from build123d import *

# Parameters (mm, degrees)
F0_W        = 31.75
F0_H        = 31.75
F1_DEPTH    = 6.35
F2_SIZE2    = 5.5380575658
F2_SIZE     = 6.6
F4_DEPTH    = 5.08
F5_T1_DEPTH = 36.3880046162
F5_T3_DEPTH = 36.3880046162


# Not quite as in the source:
# - a fillet or chamfer that OpenCascade refuses, or shapes differently, is made with other operations: its cross-section is extruded or revolved along the edge and cut away or added


with BuildPart() as f1:
    # F0 (on Top) → F1 (new body)
    with BuildSketch(Plane.XY):
        Rectangle(F0_W, F0_H)
    extrude(amount=F1_DEPTH)

    # F2
    f2_edges = [f1.edges().sort_by_distance(p)[0] for p in [
        (-15.875, 0, 6.35),
        (0, -15.875, 6.35),
        (15.875, 0, 6.35),
        (0, 15.875, 6.35),
    ]]
    f2_side = f1.faces().sort_by_distance((0, 0, 6.35))[0]
    chamfer(f2_edges, length=F2_SIZE, length2=F2_SIZE2, reference=f2_side)

    # F3 (on face) → F4 (cut)
    with BuildSketch(Plane.XY.offset(6.35)):
        with BuildLine():
            Line((9.25, -9.25), (9.25, 0))
            ThreePointArc((9.25, 0), (0, 9.25), (-9.25, 0))
            Line((-9.25, 0), (-9.25, -9.25))
            Line((-9.25, -9.25), (9.25, -9.25))
        make_face()
    extrude(amount=-F4_DEPTH, mode=Mode.SUBTRACT)

    # F5: fillet of radius 2 on 4 edges, made by hand

    # F5_s2 → F5_t1 (cut)
    with BuildSketch(Plane.YZ.offset(-18.1940023081)):
        with BuildLine():
            ThreePointArc((-15.875, 0), (-15.6643933238, 0.7771054734), (-15.1644164673, 1.4081928144))
            Line((-15.1644164673, 1.4081928144), (-15.875, 0.8119424342))
            Line((-15.875, 0.8119424342), (-15.875, 0))
        make_face()
        with BuildLine():
            ThreePointArc((15.875, 0), (15.6643933238, 0.7771054734), (15.1644164673, 1.4081928144))
            Line((15.1644164673, 1.4081928144), (15.875, 0.8119424342))
            Line((15.875, 0.8119424342), (15.875, 0))
        make_face()
    extrude(amount=F5_T1_DEPTH, mode=Mode.SUBTRACT)

    # F5_s4 → F5_t3 (cut)
    with BuildSketch(Plane.XZ.offset(-18.1940023081)):
        with BuildLine():
            ThreePointArc((15.875, 0), (15.6643933238, 0.7771054734), (15.1644164673, 1.4081928144))
            Line((15.1644164673, 1.4081928144), (15.875, 0.8119424342))
            Line((15.875, 0.8119424342), (15.875, 0))
        make_face()
        with BuildLine():
            ThreePointArc((-15.875, 0), (-15.6643933238, 0.7771054734), (-15.1644164673, 1.4081928144))
            Line((-15.1644164673, 1.4081928144), (-15.875, 0.8119424342))
            Line((-15.875, 0.8119424342), (-15.875, 0))
        make_face()
    extrude(amount=F5_T3_DEPTH, mode=Mode.SUBTRACT)


solid = f1.part
Source: CAD feature listing. Evaluate the final solid. Frame: model axes, mm. A direction names the side the tool comes from. Give positions to 0.01 mm unless a question says otherwise; leave off trailing zeros. Loops run counter-clockwise (first coordinate to the right, second up) from the corner with the lowest first, then second, coordinate; pieces in that order, holes last. Notation, with made-up numbers: (8.5, 37.5) -> (60.5, 37.5) arc R7 cw to (60.5, 44.5) -> close; hole circle Ø1 at (5, -10.5). An arc over 180 degrees is marked (long way). Use a Markdown table: item, result. Add a question column.
1) Reachability of faces 1 (the face through (-0.212, 12.261, 3.845)), 2 (the face through (0.203, 9.248, 3.846)) from +Z, -Z, +X, -X, +Y, -Y: full face, straight path, thin tool, end or side. Return the list, or none.
2) Section query D-D, the plane z = 2.25. Return the cut outline in (x, y), then the cut area to 3 significant figures.
3) Line query: line 1 along Z through (x, y) = (1, -3); line 2 along X through (y, z) = (-4, 3); line 3 along X through (y, z) = (2, 3.5). Output: solid intervals per line, ascending. Write a range as [from, to].
4) Section query B-B, the plane z = 4.5. Return the cut outline in (x, y).
5) First-contact query: pin 1 (3 mm diameter, centred on y = 5.5, z = 5.5, fed in from -X); pin 2 (9 mm diameter, centred on x = 0, y = -4.5, fed in from +Z); pin 3 (3 mm diameter, centred on x = 4.5, z = 5.5, fed in from -Y). Flat tips, straight axial feed; report the tip coordinate or a pass-through.
6) Section query A-A, the plane x = 0. Return the cut outline in (y, z) (3 decimals).
Numbers:
| question | item | result |
|---|---|---|
| 1 | face 1 | +Z, +X, -X, +Y |
| 1 | face 2 | +Z |
| 2 | outline | (-14.16, -14.16) -> (14.16, -14.16) -> (14.16, 14.16) -> (-14.16, 14.16) -> close; hole (-9.25, -9.25) -> (9.25, -9.25) -> (9.25, 0) arc R9.25 ccw to (-9.25, 0) -> close |
| 2 | area | 497 mm2 |
| 3 | line 1 | z = [0, 1.27] |
| 3 | line 2 | x = [-13.27, -9.25], [9.25, 13.27] |
| 3 | line 3 | x = [-12.67, -9.03], [9.03, 12.67] |
| 4 | outline | (-11.48, -11.48) -> (11.48, -11.48) -> (11.48, 11.48) -> (-11.48, 11.48) -> close; hole (-9.25, -9.25) -> (9.25, -9.25) -> (9.25, 0) arc R9.25 ccw to (-9.25, 0) -> close |
| 5 | pin 1 | stops at x = -12.08 |
| 5 | pin 2 | stops at z = 1.27 |
| 5 | pin 3 | stops at y = -12.08 |
| 6 | outline | (-15.875, 0) -> (15.875, 0) arc R2 ccw to (15.164, 1.408) -> (9.275, 6.35) -> (9.25, 6.35) -> (9.25, 1.27) -> (-9.25, 1.27) -> (-9.25, 6.35) -> (-9.275, 6.35) -> (-15.164, 1.408) arc R2 ccw to start |
